```python
from build123d import *

# Parameters (mm, degrees)
F0_R     = 20
F0_R_2   = 5.1
F1_DEPTH = 25
F2_R     = 6
F2_R_2   = 5.1
F3_DEPTH = 25
F4_SIZE  = 1
F5_SIZE  = 0.5


with BuildPart() as f1:
    # F0 (on Front) → F1 (new body)
    with BuildSketch(Plane.XZ):
        Circle(F0_R)
        Circle(F0_R_2, mode=Mode.SUBTRACT)
    extrude(amount=F1_DEPTH)

    # F2 (on face) → F3 (join)
    with BuildSketch(Plane(origin=(0, 0, 0), x_dir=(-1, 0, 0), z_dir=(0, 1, 0))):
        Circle(F2_R)
        Circle(F2_R_2, mode=Mode.SUBTRACT)
    extrude(amount=F3_DEPTH)

    # F4
    f4_edges = [f1.edges().sort_by_distance(p)[0] for p in [
        (-20, -25, 0),
        (-20, 0, 0),
    ]]
    chamfer(f4_edges, length=F4_SIZE)

    # F5
    f5_edges = [f1.edges().sort_by_distance(p)[0] for p in [
        (6, 25, 0),
    ]]
    chamfer(f5_edges, length=F5_SIZE)


solid = f1.part
```
Verification items for the finished model (mm, model axes). A direction names the side the tool comes from. Give positions to 0.01 mm unless a question says otherwise; leave off trailing zeros. Order: outer loops, then holes, each group sorted by start corner. A loop starts at its lowest first (then second) coordinate and runs counter-clockwise, first axis right, second up. Notation, with made-up numbers: M -26,58.5 L 26,58.5 A16 cw 26,87.5 Z; hole C -17,44 d2. An arc over 180 degrees is marked long. Answer in a Markdown table with one row per item. Add a question column.
Item 1: Section check A-A, the plane z = 0. Enter the section's corners in (x, y), and give its area (3 significant figures).
Item 2: Section check B-B, the plane x = 0. Enter the section's corners in (y, z), and give its area (3 significant figures).
Item 3: Gauge pin test, flat ends, axial feed: pin 1 (3 mm diameter, centred on x = -2.5, z = -11, fed in from +Y); pin 2 (3 mm diameter, centred on x = 0.5, y = 11.5, fed in from -Z); pin 3 (3 mm diameter, centred on y = -18.5, z = 13.5, fed in from +X). Record the tip position at first contact, or that the pin passes through.
Item 4: Section check C-C, the plane y = -21. Enter the section's corners in (x, z).
Item 5: Tool access check on faces 1 (the cylindrical face through (-4.336, -12.339, -19.524)), 2 (the flat face through (-4.5, 0, 4.5)). Record the directions out of +Z, -Z, +X, -X, +Y, -Y that give a thin tool (end or side, any length) a straight path to the whole face; none if there is none.
Item 6: Scan lines: probe 1 along Z at (x, y) = (0, 9.5); probe 2 along Z at (x, y) = (0, -14.75); probe 3 along Y at (x, z) = (2.5, -10.5). Record each from-to range of solid material in increasing order. Write a range as from..to.
Item 7: Section check D-D, the plane y = 2.5. Enter the section's corners in (x, z).
Filled sheet:
| question | item | result |
|---|---|---|
| 1 | outline | M -20,-24 L -19,-25 L -5.1,-25 L -5.1,25 L -5.5,25 L -6,24.5 L -6,0 L -19,0 L -20,-1 Z; M 5.1,-25 L 19,-25 L 20,-24 L 20,-1 L 19,0 L 6,0 L 6,24.5 L 5.5,25 L 5.1,25 Z |
| 1 | area | 788 mm^2 |
| 2 | outline | M -25,-19 L -24,-20 L -1,-20 L 0,-19 L 0,-6 L 24.5,-6 L 25,-5.5 L 25,-5.1 L -25,-5.1 Z; M -25,5.1 L 25,5.1 L 25,5.5 L 24.5,6 L 0,6 L 0,19 L -1,20 L -24,20 L -25,19 Z |
| 2 | area | 788 mm^2 |
| 3 | pin 1 | stops at y = 0 |
| 3 | pin 2 | stops at z = -6 |
| 3 | pin 3 | stops at x = 16 |
| 4 | outline | C 0,0 d40; hole C 0,0 d10.2 |
| 5 | face 1 | +Y, -Y |
| 5 | face 2 | +Y |
| 6 | probe 1 | z = -6..-5.1, 5.1..6 |
| 6 | probe 2 | z = -20..-5.1, 5.1..20 |
| 6 | probe 3 | y = -25..0 |
| 7 | outline | C 0,0 d12; hole C 0,0 d10.2 |
